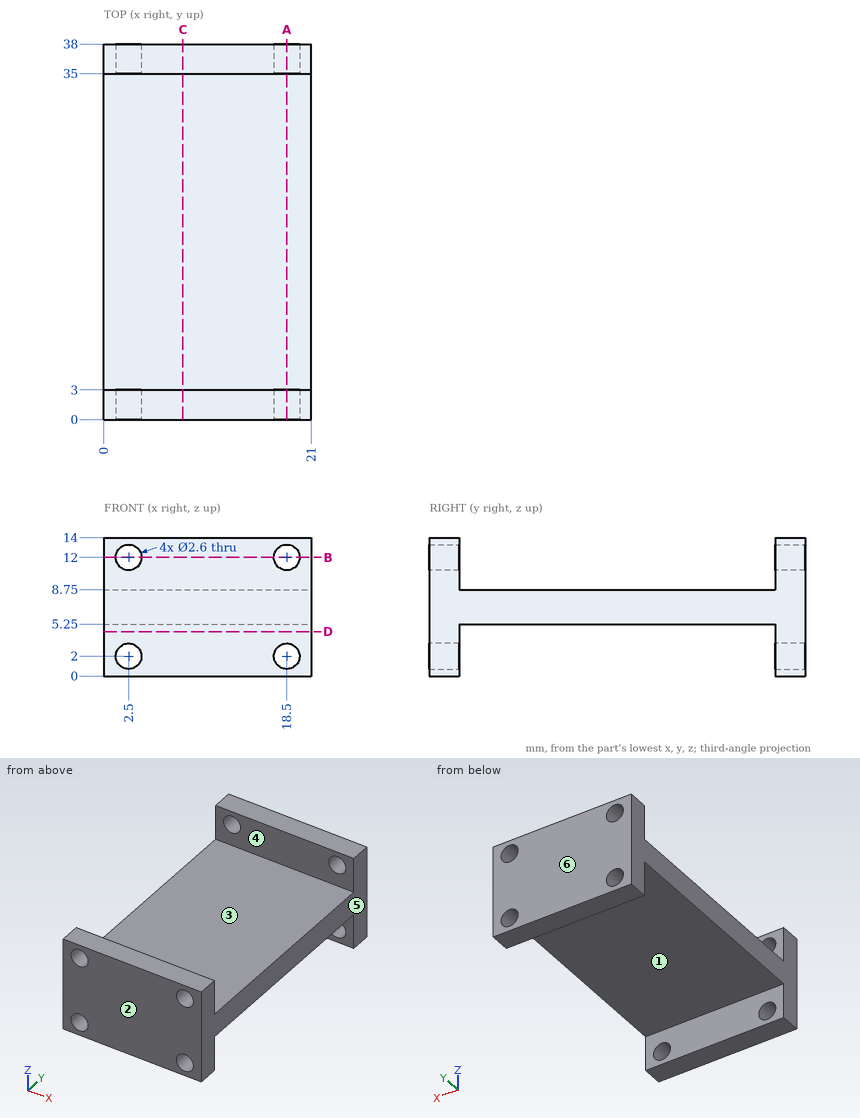
Input: dimensioned drawing with shaded views. Units: mm. Origin: part minimum x, y, z. A direction names the side the tool comes from. Coordinates: 2 decimals unless noted, no trailing zeros. Order: outer loops, then holes, each group sorted by start corner. A loop starts at its lowest first (then second) coordinate and runs counter-clockwise, first axis right, second up.
(1) Section query B-B (z = 12). Return the cut outline in (x, y), plus the area to 3 significant figures.
(2) Section query D-D (z = 4.5). Return the cut outline in (x, y), plus the area to 3 significant figures.
(3) Access query for the marked faces 1, 2 and 3. Directions: +Z, -Z, +X, -X, +Y, -Y. A direction counts if a zero-diameter tool reaches every point of the face in a straight line with its end or side. Return the directions, or none.
(4) Section query C-C (x = 8). Return the cut outline in (y, z), plus the area to 3 significant figures.
(5) Material intervals for probe 1 along X at (y, z) = (2.3, 2); probe 2 along Y at (x, z) = (17.25, 11); probe 3 along Z at (x, y) = (10.25, 34), sorted ascending.
(6) Draft query along Y for the marked faces 4, 5 and 6. Return one class per face: pulls with the +Y half, pulls with the -Y half, needs draft (parallel to the pull), parting line crosses it, or undercut.
(7) First-contact query: pin 1 (4 mm diameter, centred on x = 4, y = 17, fed in from +Z); pin 2 (1 mm diameter, centred on x = 17, y = 28, fed in from -Z). Flat tips, straight axial feed; report the tip coordinate or a pass-through.
(8) Section query A-A (x = 18.5). Return the cut outline in (y, z).
Solution:
1. outline: (0, 0) - (1.2, 0) - (1.2, 3) - (0, 3) - close; (0, 35) - (1.2, 35) - (1.2, 38) - (0, 38) - close; (3.8, 0) - (17.2, 0) - (17.2, 3) - (3.8, 3) - close; (3.8, 35) - (17.2, 35) - (17.2, 38) - (3.8, 38) - close; (19.8, 0) - (21, 0) - (21, 3) - (19.8, 3) - close; (19.8, 35) - (21, 35) - (21, 38) - (19.8, 38) - close
1. area: 94.8 mm2
2. outline: (0, 0) - (21, 0) - (21, 3) - (0, 3) - close; (0, 35) - (21, 35) - (21, 38) - (0, 38) - close
2. area: 126 mm2
3. face 1: -Z, +X, -X
3. face 2: +Z, -Z, +X, -X, -Y
3. face 3: +Z, +X, -X
4. outline: (0, 0) - (3, 0) - (3, 5.25) - (35, 5.25) - (35, 0) - (38, 0) - (38, 14) - (35, 14) - (35, 8.75) - (3, 8.75) - (3, 14) - (0, 14) - close
4. area: 196 mm2
5. probe 1: x = 0 to 1.2, 3.8 to 17.2, 19.8 to 21
5. probe 2: y = 0 to 3, 35 to 38
5. probe 3: z = 5.25 to 8.75
6. face 4: undercut
6. face 5: needs draft
6. face 6: pulls with the +Y half
7. pin 1: stops at z = 8.75
7. pin 2: stops at z = 5.25
8. outline: (0, 0) - (3, 0) - (3, 0.7) - (0, 0.7) - close; (0, 3.3) - (3, 3.3) - (3, 5.25) - (35, 5.25) - (35, 3.3) - (38, 3.3) - (38, 10.7) - (35, 10.7) - (35, 8.75) - (3, 8.75) - (3, 10.7) - (0, 10.7) - close; (0, 13.3) - (3, 13.3) - (3, 14) - (0, 14) - close; (35, 0) - (38, 0) - (38, 0.7) - (35, 0.7) - close; (35, 13.3) - (38, 13.3) - (38, 14) - (35, 14) - close
